Check sheet for the drawn part. Datum: minimum x, y, z corner. Units: mm. Coordinates: 2 decimals unless noted, no trailing zeros. Order: outer loops, then holes, each group sorted by start corner. A loop starts at its lowest first (then second) coordinate and runs counter-clockwise, first axis right, second up. Notation, with made-up numbers: (48.25, 40.5) - (67.25, 40.5) arc R30 ccw to (67.25, 71.5) - close; hole circle Ø4 at (-11.75, 12.5). An arc over 180 degrees is marked (long way). Answer as CSV lines item,"result". Start each with the question number.
1. Section check A-A (y = 0.9). Record the cut outline in (x, z).
2. Material ranges on L1, parallel to X at y = 1.2, z = 6; L2, parallel to X at y = 2.2, z = 7; L3, parallel to Z at x = 29.6, y = 1.05, recorded low to high. Write a range as [from, to].
3. Section check B-B (z = 6.6). Record the cut outline in (x, y), and give its area (3 significant figures).
4. Mould release check, pull along X, two halves, no side actions. Record for the marked faces 1, 2 and 3: pulls with the +X half, pulls with the -X half, needs draft (parallel to the pull), parting line crosses it, or undercut.
5. Section check C-C (x = 4.6). Record the cut outline in (y, z), and give its area (4 significant figures).
6. Section check D-D (x = 29.5). Record the cut outline in (y, z).
7. Go/stop test with flat-tipped pins: pin 1 (1.9 mm diameter, centred on x = 29.6, z = 6.6, fed in from -Y); pin 2 (0.9 mm diameter, centred on y = 1, z = 30, fed in from -X); pin 3 (0.9 mm diameter, centred on x = 4, y = 1.5, fed in from +Z). Record where each tip stops, or that it passes through.
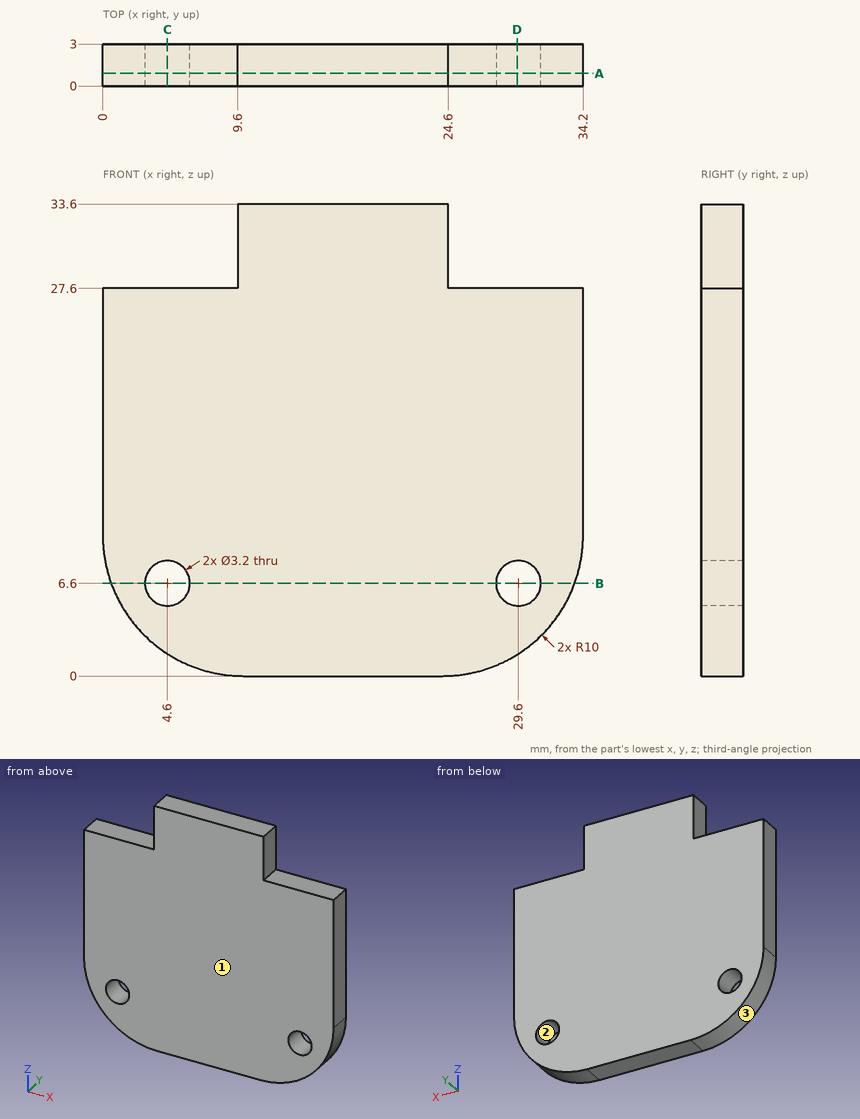
Evaluation:
1,outline,"(0, 10) arc R10 ccw to (10, 0) - (24.2, 0) arc R10 ccw to (34.2, 10) - (34.2, 27.6) - (24.6, 27.6) - (24.6, 33.6) - (9.6, 33.6) - (9.6, 27.6) - (0, 27.6) - close; hole circle Ø3.2 at (4.6, 6.6); hole circle Ø3.2 at (29.6, 6.6)"
2,L1,"x = [0.83, 3.12], [6.08, 28.12], [31.08, 33.37]"
2,L2,"x = [0.46, 3.05], [6.15, 28.05], [31.15, 33.74]"
2,L3,"z = [1.58, 5], [8.2, 27.6]"
3,outline,"(0.6, 0) - (3, 0) - (3, 3) - (0.6, 3) - close; (6.2, 0) - (28, 0) - (28, 3) - (6.2, 3) - close; (31.2, 0) - (33.6, 0) - (33.6, 3) - (31.2, 3) - close"
3,area,"79.8 mm²"
4,face 1,"needs draft"
4,face 2,"undercut"
4,face 3,"pulls with the -X half"
5,outline,"(0, 1.58) - (3, 1.58) - (3, 5) - (0, 5) - close; (0, 8.2) - (3, 8.2) - (3, 27.6) - (0, 27.6) - close"
5,area,"68.45 mm²"
6,outline,"(0, 1.52) - (3, 1.52) - (3, 5) - (0, 5) - close; (0, 8.2) - (3, 8.2) - (3, 27.6) - (0, 27.6) - close"
7,pin 1,"passes through"
7,pin 2,"stops at x = 9.6"
7,pin 3,"stops at z = 27.6"
